Source: CAD feature listing. Evaluate the final solid. Frame: model axes, mm. Face numbers are marked on the shaded views. A direction names the side the tool comes from. Coordinates: 2 decimals unless noted, no trailing zeros. Order: outer loops, then holes, each group sorted by start corner. A loop starts at its lowest first (then second) coordinate and runs counter-clockwise, first axis right, second up. Notation, with made-up numbers: (58.25, 35.25) - (113.25, 35.25) arc R11 cw to (113.25, 49.25) - close; hole circle Ø3 at (24, -23.5). An arc over 180 degrees is marked (long way). One line per question, with ' | ' between items. Start each with the question number.
(1) Section A-A (x = 0). Return the cut outline in (y, z).
(2) Access query for the marked faces 1 and 2. Directions: +Z, -Z, +X, -X, +Y, -Y. A direction counts if a zero-diameter tool reaches every point of the face in a straight line with its end or side. Return the directions, or none.
(3) Contact query for flat-ended pins moving along their axis: P1, Ø8, axis at y = 54.5, z = 2, coming from the -X side; P2, Ø1.5, axis at x = -4, y = 68.5, coming from the +Z side; P3, Ø2, axis at x = -1, y = 42, coming from the -Z side. Output: stop coordinate, or through.
(4) Section B-B (y = 131.5). Return the cut outline in (x, z).
(5) Line query: line 1 along X through (y, z) = (55.5, 3); line 2 along Y through (x, z) = (6, -1.25); line 3 along X through (y, z) = (137.5, -0.5). Output: solid intervals per line, ascending.
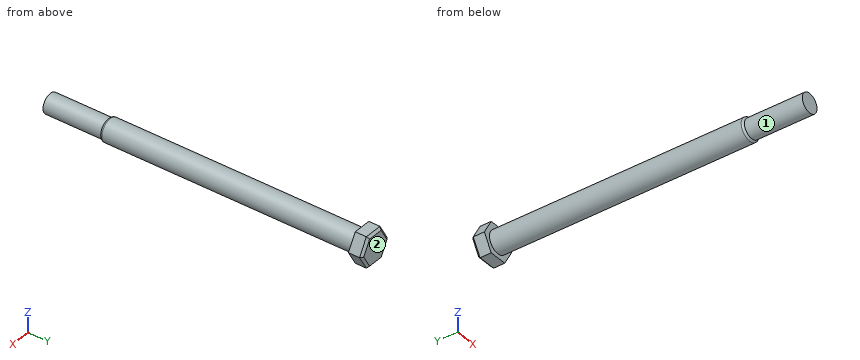
Autodesk Inventor part; units mm, degrees
ref_plane "YZ Plane" through (0, 0, 0) normal (1, 0, 0) x (0, 1, 0)
ref_plane "XZ Plane" through (0, 0, 0) normal (0, 1, 0) x (-1, 0, 0)
ref_plane "XY Plane" through (0, 0, 0) normal (0, 0, 1) x (1, 0, 0)
sketch "Sketch1" plane through (0, 0, 0) normal (0, 1, 0) x (-1, 0, 0)
  circle A0 centre (0, 0) radius 5
  dimension "d0" = 10
extrude "Extrusion1" add sketch "Sketch1" along normal blind 140
sketch "Sketch2" plane through (0, 140, 0) normal (0, 1, 0) x (1, 0, 0)
  line L0 (4, -7) -> (-4, -7)
  line L1 (-4, -7) -> (-8.0005, -0.0709)
  line L2 (-4, -7) -> (4.001, -7) construction
  line L3 (-8.0005, -0.0709) -> (-4, 6.8581)
  line L4 (-4, 6.8581) -> (4.001, 6.8581)
  line L5 (4.001, 6.8581) -> (8.0015, -0.0709)
  line L6 (8.0015, -0.0709) -> (4, -7)
  dimension "d5" = 8
  dimension "d6" = 8.001
  dimension "d7" = 120
  dimension "d8" = 8.001
  dimension "d9" = 120
  dimension "d10" = 8.001
  dimension "d11" = 120
  dimension "d12" = 8.001
  dimension "d13" = 120
extrude "Extrusion2" add sketch "Sketch2" along normal blind 6
chamfer "Chamfer1" distance 1 angle 45 6 edges at (0, 146, 7) (-6.0002, 146, 3.5355) (6.0008, 146, 3.5355) (6.0013, 146, -3.3936) (0.0005, 146, -6.8581) (-6.0002, 146, -3.3936)
sketch "Sketch3" plane through (0, 0, 0) normal (0, -1, 0) x (1, 0, 0)
  circle A0 centre (0, 0) radius 5
extrude "Extrusion3" cut sketch "Sketch3" against normal blind 26
sketch "Sketch4" plane through (0, 26, 0) normal (0, -1, 0) x (1, 0, 0)
  circle A0 centre (0, 0) radius 5
  circle A1 centre (0, 0) radius 4.3197
extrude "Extrusion4" add sketch "Sketch4" along normal blind 26 contours A1
fillet "Fillet1" radius 1 1 edges at (5, 26, 0)
thread "Thread1"
properties part number "Axel" material "Aluminum 6061-AHC"
Response values:
1) outline: (0, -4.32) - (26, -4.32) arc R1 ccw to (26.95, -5) - (140, -5) - (140, -6.86) - (145, -6.86) - (146, -5.86) - (146, 6) - (145, 7) - (140, 7) - (140, 5) - (26.95, 5) arc R1 ccw to (26, 4.32) - (0, 4.32) - close
2) face 1: -Y | face 2: +Z, -Z, +X, -X, +Y
3) P1: stops at x = -5 | P2: stops at z = 3.8 | P3: stops at z = -5
4) outline: circle Ø10 at (0, 0)
5) line 1: x = -4 to 4 | line 2: y = 140 to 146 | line 3: x = -4.97 to 4.97
